The model under review builds one solid part; all positions refer to its coordinate system, in mm. Coordinates: 2 decimals unless noted, no trailing zeros. Loops run counter-clockwise (first coordinate to the right, second up) from the corner with the lowest first, then second, coordinate; pieces in that order, holes last. Notation, with made-up numbers: M -6.5,41 L 35.5,41 A8 ccw 35.5,50 Z; hole C 56,57.25 d5. An arc over 180 degrees is marked long. Use CSV: the item, a comma, the result in double quotes. Start each with the question number.
1. For L1, parallel to X at y = 35, z = 6.5; L2, parallel to Y at x = -7.5, z = 9.75; L3, parallel to X at y = 33.5, z = 3.5, list the stretches that pass through material, from the lowest coordinate up.
2. Add section C-C, the plane x = -7.5. Write out the cut boundary in (y, z), then the cut area to 3 significant figures.
3. Draft analysis for pull direction X (two halves, no side actions). For faces 1 (the cylindrical face through (-15.21, 19.81, 8.5)), 2 (the cylindrical face through (-24.243, 33.889, 6.902)), 3 (the cylindrical face through (-29, 2, 7)), state which applies: +X half, -X half, draft (parallel to the pull), parting line (faces both ways), or undercut.
4. Clearance check with flat-ended pins moving along their axes: P1, Ø2.5, axis at x = -22.5, y = 35, coming from the -Z side; P2, Ø12, axis at x = -7, y = 13.5, coming from the -Z side; P3, Ø5, axis at x = -6, y = 17, coming from the -Z side; P4, Ø5, axis at x = -8.5, y = 21, coming from the -Z side. State where each tip first meets the part, or that it passes through.
5. Add section A-A, the plane z = 4.5. Write out the cut boundary in (x, y), then the cut area to 3 significant figures.
6. Add section D-D, the plane z = 11.25. Write out the cut boundary in (x, y), then the cut area to 3 significant figures.
7. Add section B-B, the plane y = 34. Write out the cut boundary in (x, z), then the cut area to 3 significant figures.
Autodesk Inventor part; units mm, degrees
ref_plane "YZ Plane" through (0, 0, 0) normal (1, 0, 0) x (0, 1, 0)
ref_plane "XZ Plane" through (0, 0, 0) normal (0, 1, 0) x (-1, 0, 0)
ref_plane "XY Plane" through (0, 0, 0) normal (0, 0, 1) x (1, 0, 0)
sketch "Sketch4" plane through (0, 0, 0) normal (0, 0, 1) x (1, 0, 0)
  line L0 (0, 0) -> (-30, 0)
  line L1 (-30, 0) -> (-30, 40)
  line L2 (-30, 40) -> (0, 40)
  line L3 (0, 40) -> (0, 0)
  dimension "d37" = 30
  dimension "d38" = 40
extrude "Extrusion2" add sketch "Sketch4" along normal blind 14
hole "Hole3" at (-22.5, 35, 14) direction (0, 0, -1) diameter 4.134 depth 14.2 tip angle 118
hole "Hole4" at (-7.5, 35, 14) direction (0, 0, -1) diameter 4.134 depth 14.2 tip angle 118
hole "Hole5" at (-7.5, 5, 14) direction (0, 0, -1) diameter 4.134 depth 14.2 tip angle 118
hole "Hole6" at (-22.5, 5, 14) direction (0, 0, -1) diameter 4.134 depth 14.2 tip angle 118
hole "Hole7" at (0, 20, -1) direction (-1, 0, 0) diameter 19 end through all
fillet "Fillet1" radius 5 4 edges at (-30, 40, 7) (0, 40, 7) (0, 0, 7) (-30, 0, 7)
properties part number "GARFO" material "Aluminium AW-7020"
Computed:
1,L1,"x = -30 to -24.57, -20.43 to -9.57, -5.43 to 0"
1,L2,"y = 0 to 2.93, 7.07 to 32.93, 37.07 to 40"
1,L3,"x = -30 to -23.92, -21.08 to -8.92, -6.08 to 0"
2,outline,"M 0,0 L 2.93,0 L 2.93,14 L 0,14 Z; M 7.07,0 L 10.55,0 A9.5 cw 29.45,0 L 32.93,0 L 32.93,14 L 7.07,14 Z; M 37.07,0 L 40,0 L 40,14 L 37.07,14 Z"
2,area,"321 mm^2"
3,face 1,"draft"
3,face 2,"undercut"
3,face 3,"-X half"
4,P1,"passes through"
4,P2,"stops at z = 0"
4,P3,"stops at z = 6.75"
4,P4,"stops at z = 7.83"
5,outline,"M -30,5 A5 ccw -25,0 L -5,0 A5 ccw 0,5 L 0,12.25 L -30,12.25 Z; M -30,27.75 L 0,27.75 L 0,35 A5 ccw -5,40 L -25,40 A5 ccw -30,35 Z; hole C -22.5,5 d4.13; hole C -22.5,35 d4.13; hole C -7.5,5 d4.13; hole C -7.5,35 d4.13"
5,area,"660 mm^2"
6,outline,"M -30,5 A5 ccw -25,0 L -5,0 A5 ccw 0,5 L 0,35 A5 ccw -5,40 L -25,40 A5 ccw -30,35 Z; hole C -22.5,5 d4.13; hole C -22.5,35 d4.13; hole C -7.5,5 d4.13; hole C -7.5,35 d4.13"
6,area,"1,120 mm^2"
7,outline,"M -30,0 L -24.31,0 L -24.31,14 L -30,14 Z; M -20.69,0 L -9.31,0 L -9.31,14 L -20.69,14 Z; M -5.69,0 L 0,0 L 0,14 L -5.69,14 Z"
7,area,"319 mm^2"
